The listing builds one solid part. Answer for the finished solid, in the listing's coordinates (mm). A direction names the side the tool comes from. Round coordinates to 2 decimals unless told otherwise and drop trailing zeros. Order: outer loops, then holes, each group sorted by start corner. A loop starts at its lowest first (then second) coordinate and runs counter-clockwise, first axis right, second up. Notation, with made-up numbers: (48.5, 74.25) -> (106.5, 74.25) arc R21 cw to (106.5, 112.25) -> close; hole circle Ø10 at (48.5, -12). An arc over 180 degrees is marked (long way). Return JSON: item names as keys, results as strings. Group by question number.
(1) Which of the six approach directions +Z, -Z, +X, -X, +Y, -Y give full straight-line access (tool end or side, diameter ignored) to faces 4 (the face through (-56, 1.4, 0)), 5 (the face through (-55.26, 0.71, 29.34)), 6 (the face through (53.25, 4, 0))?
(2) Each of these flat-tipped pins is pushed along its axis until it touches: pin 1 (1.6 mm diameter, centred on y = 4.5, z = 7, fed in from +X); pin 2 (4.5 mm diameter, centred on y = 4, z = 14.5, fed in from -X); pin 3 (6 mm diameter, centred on x = 57, z = 9.5, fed in from +Y); pin 4 (2 mm diameter, centred on x = -56.5, z = -25.9, fed in from +Y). Where does it stop, or does it pass through?
(3) Consider line 1 (X direction, y = 0.9, z = 29.5); line 2 (X direction, y = 5.75, z = 1.5); line 3 (Y direction, x = 34, z = 7). Determine where each line is inside the solid, lowest interval first. Write a range as [from, to].
(4) The part is cut by section C-C (z = -17). Determine the outline of the cut face in (x, y).
(5) The part is cut by section A-A (x = -56.5). Determine the outline of the cut face in (y, z), plus the area to 3 significant figures.
(6) The part is cut by section B-B (z = -25.9). Determine the outline of the cut face in (x, y).
(7) Determine the mould class of faces 1 (the face through (10, -2, 27)), 2 (the face through (57.345, 0.71, -26.821)), 3 (the face through (-1, 3, -33.75)) for opening direction Z: +Z half, -Z half, draft (parallel to the pull), parting line (faces both ways), or undercut.
(8) The part is cut by section D-D (x = 4). Determine the outline of the cut face in (y, z), plus the area to 3 significant figures.
from build123d import *

# Parameters (mm, degrees)
SKETCH_1_W          = 117.5
SKETCH_1_H          = 67.5
EXTRUDE_1_DEPTH     = 1.4
SKETCH_2_W          = 106.5
SKETCH_2_H          = 67.5
EXTRUDE_2_DEPTH     = 5.5
CUT_EXTRUDE_1_REACH = 69.977
SKETCH_5_R          = 1.25
SKETCH_6_W          = 30
SKETCH_6_H          = 6
EXTRUDE_3_DEPTH     = 2


with BuildPart() as part:
    # 草图1 → 凸台-拉伸1 (new body)
    with BuildSketch(Plane(origin=(0, 0, 0), x_dir=(1, 0, 0), z_dir=(0, 1, 0))):
        Rectangle(SKETCH_1_W, SKETCH_1_H)
    extrude(amount=EXTRUDE_1_DEPTH)

    # 草图2 → 凸台-拉伸2 (add)
    with BuildSketch(Plane(origin=(0, 1.4, 0), x_dir=(1, 0, 0), z_dir=(0, 1, 0))):
        Rectangle(SKETCH_2_W, SKETCH_2_H)
    extrude(amount=EXTRUDE_2_DEPTH)

    # 草图5 → 切除-拉伸1 (cut, up to next)
    with BuildSketch(Plane(origin=(0, 1.4, 0), x_dir=(1, 0, 0), z_dir=(0, 1, 0)), mode=Mode.PRIVATE) as cut_extrude_1_sk1:
        with Locations(Location((-56.5, -29.5, 0), (0, 0, 270))):
            Circle(SKETCH_5_R)
    cut_extrude_1_tool1 = extrude(cut_extrude_1_sk1.sketch, amount=-CUT_EXTRUDE_1_REACH, mode=Mode.PRIVATE) & part.part
    # 草图5 → 切除-拉伸1 (cut, up to next)
    with BuildSketch(Plane(origin=(0, 1.4, 0), x_dir=(1, 0, 0), z_dir=(0, 1, 0)), mode=Mode.PRIVATE) as cut_extrude_1_sk2:
        with Locations(Location((-56.5, 25.9, 0), (0, 0, 270))):
            Circle(SKETCH_5_R)
    cut_extrude_1_tool2 = extrude(cut_extrude_1_sk2.sketch, amount=-CUT_EXTRUDE_1_REACH, mode=Mode.PRIVATE) & part.part
    # 草图5 → 切除-拉伸1 (cut, up to next)
    with BuildSketch(Plane(origin=(0, 1.4, 0), x_dir=(1, 0, 0), z_dir=(0, 1, 0)), mode=Mode.PRIVATE) as cut_extrude_1_sk3:
        with Locations(Location((56.5, 25.9, 0), (0, 0, 270))):
            Circle(SKETCH_5_R)
    cut_extrude_1_tool3 = extrude(cut_extrude_1_sk3.sketch, amount=-CUT_EXTRUDE_1_REACH, mode=Mode.PRIVATE) & part.part
    # 草图5 → 切除-拉伸1 (cut, up to next)
    with BuildSketch(Plane(origin=(0, 1.4, 0), x_dir=(1, 0, 0), z_dir=(0, 1, 0)), mode=Mode.PRIVATE) as cut_extrude_1_sk4:
        with Locations(Location((56.5, -29.5, 0), (0, 0, 270))):
            Circle(SKETCH_5_R)
    cut_extrude_1_tool4 = extrude(cut_extrude_1_sk4.sketch, amount=-CUT_EXTRUDE_1_REACH, mode=Mode.PRIVATE) & part.part
    add(cut_extrude_1_tool1.solids().sort_by_distance((-56.5, 1.4, 29.5))[0], mode=Mode.SUBTRACT)
    add(cut_extrude_1_tool2.solids().sort_by_distance((-56.5, 1.4, -25.9))[0], mode=Mode.SUBTRACT)
    add(cut_extrude_1_tool3.solids().sort_by_distance((56.5, 1.4, -25.9))[0], mode=Mode.SUBTRACT)
    add(cut_extrude_1_tool4.solids().sort_by_distance((56.5, 1.4, 29.5))[0], mode=Mode.SUBTRACT)

    # 草图6 → 凸台-拉伸3 (add)
    with BuildSketch(Plane.XZ):
        with Locations((10.25, 27.25)):
            Rectangle(SKETCH_6_W, SKETCH_6_H)
    extrude(amount=EXTRUDE_3_DEPTH)


solid = part.part
Answer below:
{
 "1": {"face 4": "+Z, -Z, -X, +Y", "face 5": "+Y, -Y", "face 6": "+Z, -Z, +X, +Y"},
 "2": {"pin 1": "stops at x = 53.25", "pin 2": "stops at x = -53.25", "pin 3": "stops at y = 1.4", "pin 4": "passes through"},
 "3": {"line 1": "x = [-58.75, -57.75], [-55.25, 55.25], [57.75, 58.75]", "line 2": "x = [-53.25, 53.25]", "line 3": "y = [0, 6.9]"},
 "4": {"outline": "(-58.75, 0) -> (58.75, 0) -> (58.75, 1.4) -> (53.25, 1.4) -> (53.25, 6.9) -> (-53.25, 6.9) -> (-53.25, 1.4) -> (-58.75, 1.4) -> close"},
 "5": {"outline": "(0, -33.75) -> (1.4, -33.75) -> (1.4, -27.15) -> (0, -27.15) -> close; (0, -24.65) -> (1.4, -24.65) -> (1.4, 28.25) -> (0, 28.25) -> close; (0, 30.75) -> (1.4, 30.75) -> (1.4, 33.75) -> (0, 33.75) -> close", "area": "87.5 mm²"},
 "6": {"outline": "(-58.75, 0) -> (-57.75, 0) -> (-57.75, 1.4) -> (-58.75, 1.4) -> close; (-55.25, 0) -> (55.25, 0) -> (55.25, 1.4) -> (53.25, 1.4) -> (53.25, 6.9) -> (-53.25, 6.9) -> (-53.25, 1.4) -> (-55.25, 1.4) -> close; (57.75, 0) -> (58.75, 0) -> (58.75, 1.4) -> (57.75, 1.4) -> close"},
 "7": {"face 1": "draft", "face 2": "undercut", "face 3": "-Z half"},
 "8": {"outline": "(-2, 24.25) -> (0, 24.25) -> (0, -33.75) -> (6.9, -33.75) -> (6.9, 33.75) -> (0, 33.75) -> (0, 30.25) -> (-2, 30.25) -> close", "area": "478 mm²"}
}
